The figure shows three views and two pictorial views of one solid part (mm, origin at its lowest corner). Answer the questions. A direction names the side the tool comes from. Coordinates: 2 decimals unless noted, no trailing zeros. Loops run counter-clockwise (first coordinate to the right, second up) from the corner with the lowest first, then second, coordinate; pieces in that order, holes last. Notation, with made-up numbers: M -33.75,76.25 L -22.75,76.25 A25 ccw -22.75,108.25 Z; hole C 60.25,69.25 d1. An arc over 180 degrees is marked long. Answer as a JSON object with one key per item and string values. Group by question number.
1. Given pin 1 (8 mm diameter, centred on y = 7, z = 121, fed in from -X); pin 2 (3 mm diameter, centred on x = 55.5, y = 13, fed in from -Z); pin 3 (9 mm diameter, centred on y = 21, z = 142, fed in from +X); pin 4 (10.5 mm diameter, centred on x = 29.5, z = 160, fed in from +Y), each flat-ended and moving along its own axis, determine where each tip first touches the part or whether it passes through.
2. Straight lines are drawn through the part: L1, parallel to X at y = 24.25, z = 120.5; L2, parallel to Z at x = 28, y = 4.25; L3, parallel to X at y = 7.25, z = 99. For each, find the intervals that lie inside material, in ascending order.
3. A cutting plane is placed at B-B on x = 14. Give the vertices of the cut face in (y, z), and give its area (3 significant figures).
4. A cutting plane is placed at C-C on y = 25.5. Give the vertices of the cut face in (x, z).
5. For the marked faces 1, 2 and 3, determine the directions among +Z, -Z, +X, -X, +Y, -Y from which every point of the face is accessible in a straight line to the end or side of a thin tool.
6. A cutting plane is placed at A-A on z = 84.5. Give the vertices of the cut face in (x, y).
7. A cutting plane is placed at D-D on y = 2.25. Give the vertices of the cut face in (x, z), and give its area (3 significant figures).
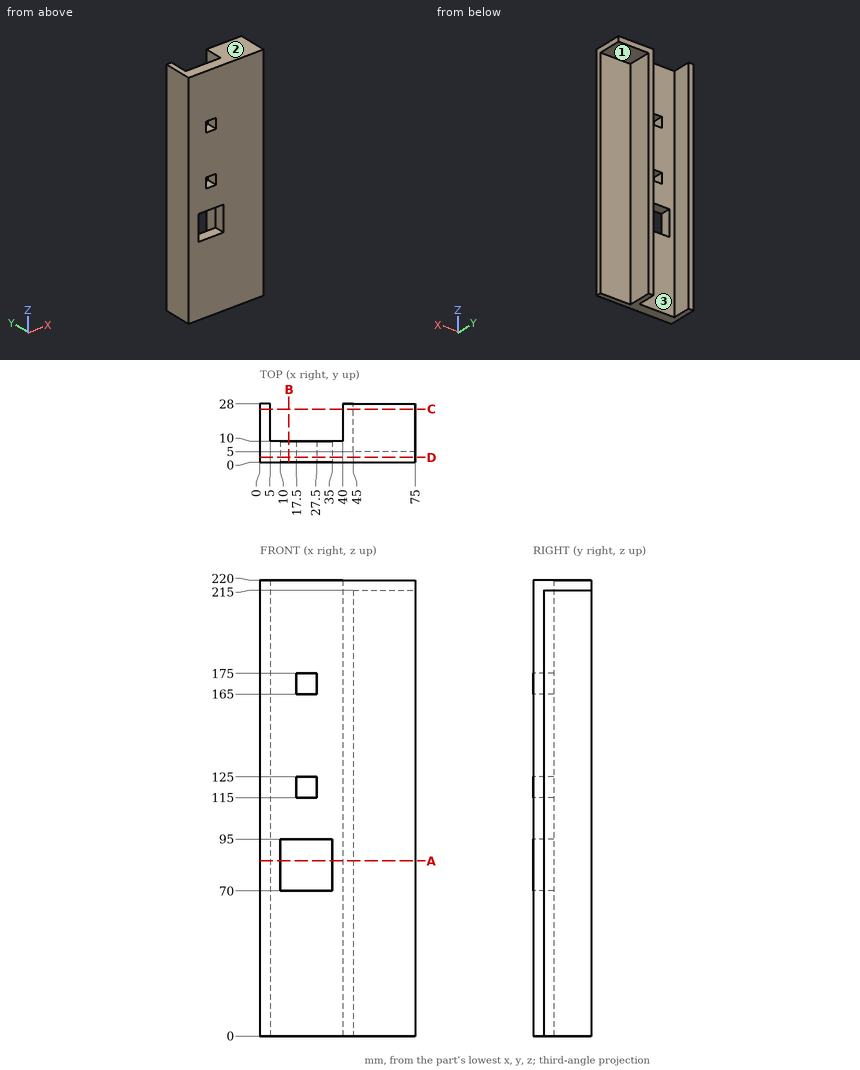
From the geometry:
{
 "1": {"pin 1": "stops at x = 0", "pin 2": "stops at z = 215", "pin 3": "stops at x = 45", "pin 4": "stops at y = 10"},
 "2": {"L1": "x = 0 to 5, 40 to 45", "L2": "z = 0 to 70, 95 to 220", "L3": "x = 0 to 45"},
 "3": {"outline": "M 0,0 L 10,0 L 10,70 L 0,70 Z; M 0,95 L 10,95 L 10,220 L 0,220 Z", "area": "1,950 mm²"},
 "4": {"outline": "M 0,0 L 5,0 L 5,220 L 0,220 Z; M 40,0 L 45,0 L 45,215 L 75,215 L 75,220 L 40,220 Z"},
 "5": {"face 1": "-Z, +X, +Y", "face 2": "+Z, +X, -X, +Y, -Y", "face 3": "+Z, -Z, +Y"},
 "6": {"outline": "M 0,0 L 10,0 L 10,10 L 5,10 L 5,28 L 0,28 Z; M 35,0 L 75,0 L 75,5 L 45,5 L 45,28 L 40,28 L 40,10 L 35,10 Z"},
 "7": {"outline": "M 0,0 L 75,0 L 75,220 L 0,220 Z; hole M 10,70 L 35,70 L 35,95 L 10,95 Z; hole M 17.5,115 L 27.5,115 L 27.5,125 L 17.5,125 Z; hole M 17.5,165 L 27.5,165 L 27.5,175 L 17.5,175 Z", "area": "15,700 mm²"}
}
